Design review of the part shown in the three views and the two pictorial views. Dimensions are in mm from the part's minimum x, y and z. A direction names the side the tool comes from. Round coordinates to 2 decimals unless told otherwise and drop trailing zeros. Order: outer loops, then holes, each group sorted by start corner. A loop starts at its lowest first (then second) coordinate and runs counter-clockwise, first axis right, second up. Notation, with made-up numbers: (76, -18.5) -> (134, -18.5) arc R33 cw to (134, 16.5) -> close; hole circle Ø4 at (-36, -29.75). An arc over 180 degrees is marked (long way). Put each result on its own line as item: value. Start each with the question number.
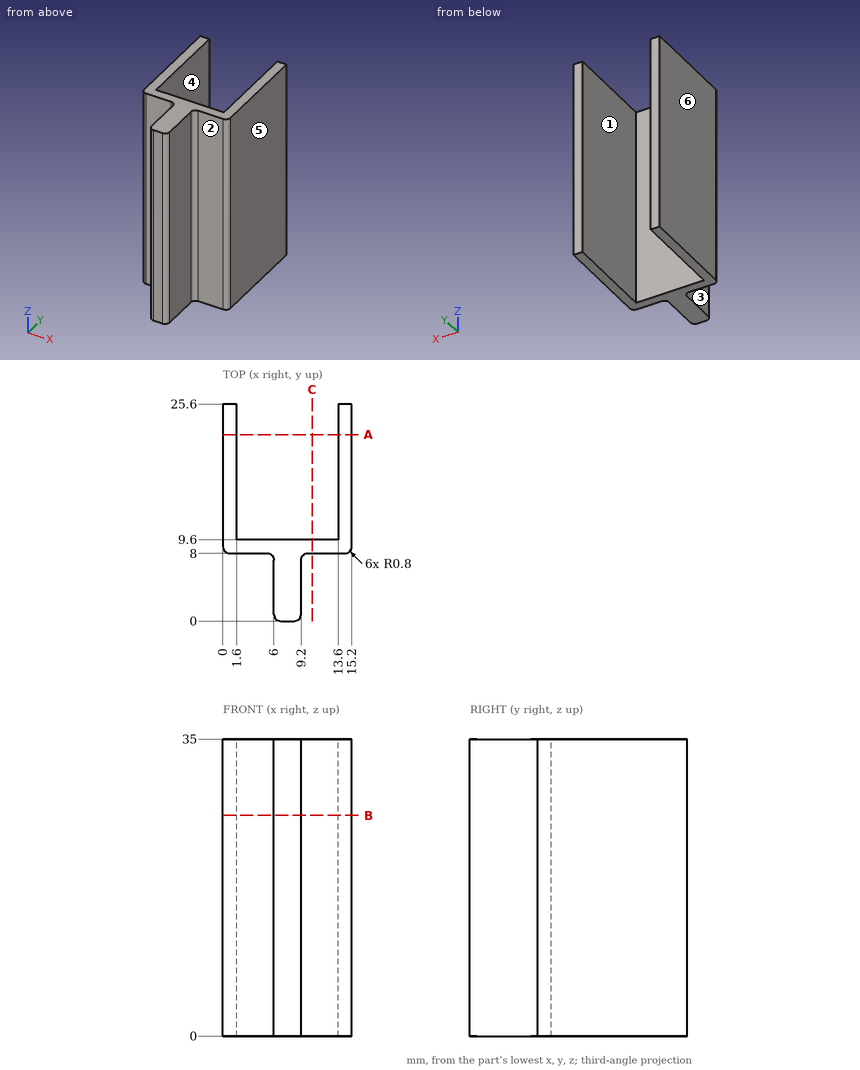
Q1. For the marked faces 1, 2 and 3, list the 3-axis set-ups (+Z, -Z, +X, -X, +Y, -Y) from which the entire face can be reached by the end or side of a thin tool; tool diameter is ignored.
Q2. Take a section at A-A on y = 22. Give the boundary of the cut face in (x, z), and give its area (3 significant figures).
Q3. Draft analysis for pull direction X (two halves, no side actions). For the marked faces 4, 5 and 6, state which applies: +X half, -X half, draft (parallel to the pull), parting line (faces both ways), or undercut.
Q4. Take a section at B-B on z = 26. Give the boundary of the cut face in (x, y), and give its area (3 significant figures).
Q5. Take a section at C-C on x = 10.5. Give the boundary of the cut face in (y, z), and give its area (3 significant figures).
Q6. Clearance check with flat-ended pins moving along their axes: pin 1 Ø3.5 at (x, z) = (3, 15.5) entering from -Y; pin 2 Ø1.9 at (y, z) = (4.5, 15.5) entering from -X; pin 3 Ø3.5 at (x, z) = (5, 17) entering from +Y. State where each tip first meets the part, or that it passes through.
Q7. Wall thickness on probe 1 along X at (y, z) = (19.5, 32.5); probe 2 along Y at (x, z) = (3.5, 2.5); probe 3 along Y at (x, z) = (7.25, 28.5): over which ranges is each line inside the solid? List them lowest first. Write a range as [from, to].
Calculated:
1. face 1: +Z, -Z, +Y
1. face 2: +Z, -Z, +X, -Y
1. face 3: +Z, -Z, -X, -Y
2. outline: (0, 0) -> (1.6, 0) -> (1.6, 35) -> (0, 35) -> close; (13.6, 0) -> (15.2, 0) -> (15.2, 35) -> (13.6, 35) -> close
2. area: 112 mm²
3. face 4: undercut
3. face 5: +X half
3. face 6: -X half
4. outline: (0, 8.8) arc R0.8 ccw to (0.8, 8) -> (5.2, 8) arc R0.8 cw to (6, 7.2) -> (6, 0.8) arc R0.8 ccw to (6.8, 0) -> (8.4, 0) arc R0.8 ccw to (9.2, 0.8) -> (9.2, 7.2) arc R0.8 cw to (10, 8) -> (14.4, 8) arc R0.8 ccw to (15.2, 8.8) -> (15.2, 25.6) -> (13.6, 25.6) -> (13.6, 9.6) -> (1.6, 9.6) -> (1.6, 25.6) -> (0, 25.6) -> close
4. area: 101 mm²
5. outline: (8, 0) -> (9.6, 0) -> (9.6, 35) -> (8, 35) -> close
5. area: 56.0 mm²
6. pin 1: stops at y = 8
6. pin 2: stops at x = 6
6. pin 3: stops at y = 9.6
7. probe 1: x = [0, 1.6], [13.6, 15.2]
7. probe 2: y = [8, 9.6]
7. probe 3: y = [0, 9.6]
